Design review of the part built by this model. Coordinates are the model's own, in mm. A direction names the side the tool comes from. Coordinates: 2 decimals unless noted, no trailing zeros.
Q1. Insertion check: pin 1 (4 mm diameter, centred on y = 11, z = 6, fed in from -X); pin 2 (2 mm diameter, centred on y = -1, z = 15.5, fed in from +X); pin 3 (8 mm diameter, centred on x = 9.5, z = 9.5, fed in from +Y). Each pin has a flat end and moves straight along its axis. Give the tip position at first contact, or say it passes through.
Q2. Mouldability with a two-part tool opening along X and no side actions: class faces 6 (the cylindrical face through (3.8, 14.28, 11.09)), 7 (the flat face through (-9.674, 9.004, 11.092)), 8 (the cylindrical face through (-7.41, 12.783, 11.092)) as pulls with the +X half, pulls with the -X half, needs draft (parallel to the pull), parting line crosses it, or undercut.
Q3. For probe 1 along Z at (x, y) = (7.5, -11.75); probe 2 along Y at (x, z) = (2.5, 7); probe 3 along Y at (x, z) = (12.25, 15.25), list the stretches that pass through material, from the lowest coordinate up.
Q4. Machinability: for faces 1 (the flat face through (3.521, 0, 9)), 2 (the cylindrical face through (11.3, 3.9, 11.1)), 3 (the flat face through (-12.8, -3, 11.1)), 4 (the cylindrical face through (1.19, -5.37, -4.12)), 5 (the cylindrical face through (-14.645, -1.954, 11.092)), which of the approach directions +Z, -Z, +X, -X, +Y, -Y give a long, thin tool a straight path to every point of the face, cutting with its end or side? Answer none if there is none.
```python
from build123d import *

# Parameters (mm, degrees)
SALIENTE_EXTRUIR1_DEPTH    = 15
CROQUIS5_R                 = 4.5
SALIENTE_EXTRUIR2_DEPTH    = 6
ESCALA1_SCALE              = 1.5
CORTAR_EXTRUIR3_DEPTH      = 38.7502155
CORTAR_EXTRUIR3_DEPTH_BACK = 5.8
CROQUIS7_R                 = 10
CROQUIS8_R                 = 5.5
SALIENTE_EXTRUIR3_DEPTH    = 1.87
CORTAR_EXTRUIR4_DEPTH      = 35.538871873
CORTAR_EXTRUIR4_DEPTH_BACK = 35.538871873


with BuildPart() as part:
    # Croquis2 → Saliente-Extruir1 (new body)
    with BuildSketch(Plane.XY):
        with BuildLine():
            Line((-2.081696937, 7.693567449), (-1.911179214, 9.445287663))
            ThreePointArc((-1.911179214, 9.445287663), (-1.831468139, 9.618345927), (-1.663611198, 9.708496165))
            ThreePointArc((-1.663611198, 9.708496165), (-1.297642615, 9.764149919), (-0.929841298, 9.806013214))
            ThreePointArc((-0.929841298, 9.806013214), (-0.744265019, 9.762833784), (-0.622120698, 9.616601835))
            Line((-0.622120698, 9.616601835), (0, 7.97022222))
            ThreePointArc((0, 7.97022222), (0.511536449, 7.953789832), (1.020963606, 7.904560428))
            Line((1.020963606, 7.904560428), (1.848855744, 9.457684572))
            ThreePointArc((1.848855744, 9.457684572), (1.988725705, 9.587065453), (2.1783043, 9.606117341))
            ThreePointArc((2.1783043, 9.606117341), (2.537712953, 9.517484592), (2.893537451, 9.415409764))
            ThreePointArc((2.893537451, 9.415409764), (3.048463524, 9.304500205), (3.105349619, 9.122656892))
            Line((3.105349619, 9.122656892), (3.050071996, 7.363525179))
            ThreePointArc((3.050071996, 7.363525179), (3.516381649, 7.152587108), (3.968191694, 6.912155736))
            Line((3.968191694, 6.912155736), (5.327419174, 8.030234739))
            ThreePointArc((5.327419174, 8.030234739), (5.506154088, 8.09624117), (5.688592714, 8.041294232))
            ThreePointArc((5.688592714, 8.041294232), (5.986724728, 7.821868513), (6.276401353, 7.591395527))
            ThreePointArc((6.276401353, 7.591395527), (6.37709113, 7.429640815), (6.360058606, 7.239870134))
            Line((6.360058606, 7.239870134), (5.635798179, 5.635798179))
            ThreePointArc((5.635798179, 5.635798179), (5.985889619, 5.262467835), (6.311298569, 4.867437992))
            Line((6.311298569, 4.867437992), (7.994931329, 5.380254461))
            ThreePointArc((7.994931329, 5.380254461), (8.185320425, 5.372837562), (8.332844455, 5.252256971))
            ThreePointArc((8.332844455, 5.252256971), (8.524311933, 4.935443857), (8.703740045, 4.611660138))
            ThreePointArc((8.703740045, 4.611660138), (8.73486442, 4.42368596), (8.646506324, 4.254878777))
            Line((8.646506324, 4.254878777), (7.363525179, 3.050071996))
            ThreePointArc((7.363525179, 3.050071996), (7.544100156, 2.571185538), (7.693567449, 2.081696937))
            Line((7.693567449, 2.081696937), (9.445287663, 1.911179214))
            ThreePointArc((9.445287663, 1.911179214), (9.618345927, 1.831468139), (9.708496165, 1.663611198))
            ThreePointArc((9.708496165, 1.663611198), (9.764149919, 1.297642615), (9.806013214, 0.929841298))
            ThreePointArc((9.806013214, 0.929841298), (9.762833784, 0.744265019), (9.616601835, 0.622120698))
            Line((9.616601835, 0.622120698), (7.97022222, 0))
            ThreePointArc((7.97022222, 0), (7.953789832, -0.511536449), (7.904560428, -1.020963606))
            Line((7.904560428, -1.020963606), (9.457684572, -1.848855744))
            ThreePointArc((9.457684572, -1.848855744), (9.587065453, -1.988725705), (9.606117341, -2.1783043))
            ThreePointArc((9.606117341, -2.1783043), (9.517484592, -2.537712953), (9.415409764, -2.893537451))
            ThreePointArc((9.415409764, -2.893537451), (9.304500205, -3.048463524), (9.122656892, -3.105349619))
            Line((9.122656892, -3.105349619), (7.363525179, -3.050071996))
            ThreePointArc((7.363525179, -3.050071996), (7.152587108, -3.516381649), (6.912155736, -3.968191694))
            Line((6.912155736, -3.968191694), (8.030234739, -5.327419174))
            ThreePointArc((8.030234739, -5.327419174), (8.09624117, -5.506154088), (8.041294232, -5.688592714))
            ThreePointArc((8.041294232, -5.688592714), (7.821868513, -5.986724728), (7.591395527, -6.276401353))
            ThreePointArc((7.591395527, -6.276401353), (7.429640815, -6.37709113), (7.239870134, -6.360058606))
            Line((7.239870134, -6.360058606), (5.635798179, -5.635798179))
            ThreePointArc((5.635798179, -5.635798179), (5.262467835, -5.985889619), (4.867437992, -6.311298569))
            Line((4.867437992, -6.311298569), (5.380254461, -7.994931329))
            ThreePointArc((5.380254461, -7.994931329), (5.372837562, -8.185320425), (5.252256971, -8.332844455))
            ThreePointArc((5.252256971, -8.332844455), (4.935443857, -8.524311933), (4.611660138, -8.703740045))
            ThreePointArc((4.611660138, -8.703740045), (4.42368596, -8.73486442), (4.254878777, -8.646506324))
            Line((4.254878777, -8.646506324), (3.050071996, -7.363525179))
            ThreePointArc((3.050071996, -7.363525179), (2.571185538, -7.544100156), (2.081696937, -7.693567449))
            Line((2.081696937, -7.693567449), (1.911179214, -9.445287663))
            ThreePointArc((1.911179214, -9.445287663), (1.831468139, -9.618345927), (1.663611198, -9.708496165))
            ThreePointArc((1.663611198, -9.708496165), (1.297642615, -9.764149919), (0.929841298, -9.806013214))
            ThreePointArc((0.929841298, -9.806013214), (0.744265019, -9.762833784), (0.622120698, -9.616601835))
            Line((0.622120698, -9.616601835), (0, -7.97022222))
            ThreePointArc((0, -7.97022222), (-0.511536449, -7.953789832), (-1.020963606, -7.904560428))
            Line((-1.020963606, -7.904560428), (-1.848855744, -9.457684572))
            ThreePointArc((-1.848855744, -9.457684572), (-1.988725705, -9.587065453), (-2.1783043, -9.606117341))
            ThreePointArc((-2.1783043, -9.606117341), (-2.537712953, -9.517484592), (-2.893537451, -9.415409764))
            ThreePointArc((-2.893537451, -9.415409764), (-3.048463524, -9.304500205), (-3.105349619, -9.122656892))
            Line((-3.105349619, -9.122656892), (-3.050071996, -7.363525179))
            ThreePointArc((-3.050071996, -7.363525179), (-3.516381649, -7.152587108), (-3.968191694, -6.912155736))
            Line((-3.968191694, -6.912155736), (-5.327419174, -8.030234739))
            ThreePointArc((-5.327419174, -8.030234739), (-5.506154088, -8.09624117), (-5.688592714, -8.041294232))
            ThreePointArc((-5.688592714, -8.041294232), (-5.986724728, -7.821868513), (-6.276401353, -7.591395527))
            ThreePointArc((-6.276401353, -7.591395527), (-6.37709113, -7.429640815), (-6.360058606, -7.239870134))
            Line((-6.360058606, -7.239870134), (-5.635798179, -5.635798179))
            ThreePointArc((-5.635798179, -5.635798179), (-5.985889619, -5.262467835), (-6.311298569, -4.867437992))
            Line((-6.311298569, -4.867437992), (-7.994931329, -5.380254461))
            ThreePointArc((-7.994931329, -5.380254461), (-8.185320425, -5.372837562), (-8.332844455, -5.252256971))
            ThreePointArc((-8.332844455, -5.252256971), (-8.524311933, -4.935443857), (-8.703740045, -4.611660138))
            ThreePointArc((-8.703740045, -4.611660138), (-8.73486442, -4.42368596), (-8.646506324, -4.254878777))
            Line((-8.646506324, -4.254878777), (-7.363525179, -3.050071996))
            ThreePointArc((-7.363525179, -3.050071996), (-7.544100156, -2.571185538), (-7.693567449, -2.081696937))
            Line((-7.693567449, -2.081696937), (-9.445287663, -1.911179214))
            ThreePointArc((-9.445287663, -1.911179214), (-9.618345927, -1.831468139), (-9.708496165, -1.663611198))
            ThreePointArc((-9.708496165, -1.663611198), (-9.764149919, -1.297642615), (-9.806013214, -0.929841298))
            ThreePointArc((-9.806013214, -0.929841298), (-9.762833784, -0.744265019), (-9.616601835, -0.622120698))
            Line((-9.616601835, -0.622120698), (-7.97022222, 0))
            ThreePointArc((-7.97022222, 0), (-7.953789832, 0.511536449), (-7.904560428, 1.020963606))
            Line((-7.904560428, 1.020963606), (-9.457684572, 1.848855744))
            ThreePointArc((-9.457684572, 1.848855744), (-9.587065453, 1.988725705), (-9.606117341, 2.1783043))
            ThreePointArc((-9.606117341, 2.1783043), (-9.517484592, 2.537712953), (-9.415409764, 2.893537451))
            ThreePointArc((-9.415409764, 2.893537451), (-9.304500205, 3.048463524), (-9.122656892, 3.105349619))
            Line((-9.122656892, 3.105349619), (-7.363525179, 3.050071996))
            ThreePointArc((-7.363525179, 3.050071996), (-7.152587108, 3.516381649), (-6.912155736, 3.968191694))
            Line((-6.912155736, 3.968191694), (-8.030234739, 5.327419174))
            ThreePointArc((-8.030234739, 5.327419174), (-8.09624117, 5.506154088), (-8.041294232, 5.688592714))
            ThreePointArc((-8.041294232, 5.688592714), (-7.821868513, 5.986724728), (-7.591395527, 6.276401353))
            ThreePointArc((-7.591395527, 6.276401353), (-7.429640815, 6.37709113), (-7.239870134, 6.360058606))
            Line((-7.239870134, 6.360058606), (-5.635798179, 5.635798179))
            ThreePointArc((-5.635798179, 5.635798179), (-5.262467835, 5.985889619), (-4.867437992, 6.311298569))
            Line((-4.867437992, 6.311298569), (-5.380254461, 7.994931329))
            ThreePointArc((-5.380254461, 7.994931329), (-5.372837562, 8.185320425), (-5.252256971, 8.332844455))
            ThreePointArc((-5.252256971, 8.332844455), (-4.935443857, 8.524311933), (-4.611660138, 8.703740045))
            ThreePointArc((-4.611660138, 8.703740045), (-4.42368596, 8.73486442), (-4.254878777, 8.646506324))
            Line((-4.254878777, 8.646506324), (-3.050071996, 7.363525179))
            ThreePointArc((-3.050071996, 7.363525179), (-2.571185538, 7.544100156), (-2.081696937, 7.693567449))
        make_face()
    extrude(amount=SALIENTE_EXTRUIR1_DEPTH)

    # Croquis5 → Saliente-Extruir2 (add)
    with BuildSketch(Plane(origin=(0, 0, 0), x_dir=(-1, 0, 0), z_dir=(0, 0, -1))):
        with Locations(Location((0, 0, 0), (0, 0, 180))):
            Circle(CROQUIS5_R)
    extrude(amount=SALIENTE_EXTRUIR2_DEPTH)


with BuildPart() as part_1:
    # Escala1: scaled about (0, 0, 0)
    add(part.part.scale(ESCALA1_SCALE))

    # Croquis7 → Cortar-Extruir3 (cut, two sides: drawn at the far end of the back side and taken through both)
    with BuildSketch(Plane(origin=(0, 0, -9), x_dir=(-1, 0, 0), z_dir=(0, 0, -1)).offset(-CORTAR_EXTRUIR3_DEPTH_BACK)):
        Circle(CROQUIS7_R)
    extrude(amount=CORTAR_EXTRUIR3_DEPTH + CORTAR_EXTRUIR3_DEPTH_BACK, mode=Mode.SUBTRACT)

    # Croquis8 → Saliente-Extruir3 (add)
    with BuildSketch(Plane(origin=(0, 0, -3.2), x_dir=(-1, 0, 0), z_dir=(0, 0, -1))):
        Circle(CROQUIS8_R)
    extrude(amount=SALIENTE_EXTRUIR3_DEPTH)

    # Croquis10 → Cortar-Extruir4 (cut, two sides: drawn at the far end of the back side and taken through both)
    with BuildSketch(Plane.XY.offset(22.5).offset(-CORTAR_EXTRUIR4_DEPTH_BACK)):
        Polygon((0, 4.065470054), (-3.520800345, 2.032735027), (-3.520800345, -2.032735027), (0, -4.065470054), (3.520800345, -2.032735027), (3.520800345, 2.032735027), align=None)
    extrude(amount=CORTAR_EXTRUIR4_DEPTH + CORTAR_EXTRUIR4_DEPTH_BACK, mode=Mode.SUBTRACT)


solid = part_1.part
```
Response:
1. pin 1: stops at x = -11.72
1. pin 2: stops at x = 12.74
1. pin 3: stops at y = 12.14
2. face 6: pulls with the +X half
2. face 7: undercut
2. face 8: pulls with the -X half
3. probe 1: z = 0 to 22.5
3. probe 2: y = -14.56 to -2.62, 2.62 to 13.67
3. probe 3: y = -4.61 to -1.74, 0.11 to 3.05, 5.71 to 8.07
4. face 1: +Z, -Z
4. face 2: +Z, -Z, +X
4. face 3: +Z, -Z, -X
4. face 4: -Z
4. face 5: +Z, -Z, -X, -Y
